Build history of the part. All positions in model axes, mm. A direction names the side the tool comes from. Give positions to 0.01 mm unless a question says otherwise; leave off trailing zeros. Loops run counter-clockwise (first coordinate to the right, second up) from the corner with the lowest first, then second, coordinate; pieces in that order, holes last. Notation, with made-up numbers: M 9,-26.5 L 32,-26.5 A12 ccw 32,-7.5 Z; hole C 13.25,86 d3. An arc over 180 degrees is marked long. Answer in a Markdown table with one row per item. Add a question column.
```python
from build123d import *

# Parameters (mm, degrees)
SKETCH1_W           = 48
SKETCH1_H           = 48
BOSS_EXTRUDE1_DEPTH = 60
SKETCH2_W           = 48
SKETCH2_H           = 48
BOSS_EXTRUDE2_DEPTH = 25
FILLET1_R           = 24
SKETCH3_R           = 5
BOSS_EXTRUDE3_DEPTH = 10
SKETCH4_R           = 5
CUT_EXTRUDE1_DEPTH  = 15
SKETCH5_W           = 31.72674495
SKETCH5_H           = 26.264357258
CUT_EXTRUDE2_DEPTH  = 2
SKETCH8_W           = 31.72674495
SKETCH8_H           = 26.264357258
BOSS_EXTRUDE6_DEPTH = 1
FILLET3_R           = 1.5


# Some blends are built 0.0001 mm under size
with BuildPart() as part:
    # Sketch1 → Boss-Extrude1 (new body)
    with BuildSketch(Plane(origin=(0, 0, 0), x_dir=(1, 0, 0), z_dir=(0, 1, 0))):
        with Locations((24, 24)):
            Rectangle(SKETCH1_W, SKETCH1_H)
    extrude(amount=BOSS_EXTRUDE1_DEPTH)

    # Sketch2 → Boss-Extrude2 (add)
    with BuildSketch(Plane(origin=(48, 0, 0), x_dir=(0, 0, -1), z_dir=(1, 0, 0))):
        with Locations((24, 31.5)):
            Rectangle(SKETCH2_W, SKETCH2_H)
    extrude(amount=BOSS_EXTRUDE2_DEPTH)

    # Fillet1
    fillet1_edges = [part.edges().sort_by_distance(p)[0] for p in [
        (0, 30, 0),
        (0, 30, -48),
        (48, 57.75, -48),
        (48, 57.75, 0),
        (48, 3.75, -48),
        (48, 3.75, 0),
        (60.5, 7.5, 0),
        (60.5, 55.5, 0),
        (60.5, 7.5, -48),
        (60.5, 55.5, -48),
    ]]
    fillet(fillet1_edges, radius=FILLET1_R - 0.0001)  # a hair under: the kernel refuses the full size

    # Sketch3 → Boss-Extrude3 (add)
    with BuildSketch(Plane(origin=(0, 0, 0), x_dir=(-1, 0, 0), z_dir=(0, -1, 0))):
        with Locations(Location((-24, 24, 0), (0, 0, 90))):
            Circle(SKETCH3_R)
    extrude(amount=BOSS_EXTRUDE3_DEPTH)

    # Sketch4 → Cut-Extrude1 (cut)
    with BuildSketch(Plane(origin=(73, 0, 0), x_dir=(0, 0, -1), z_dir=(1, 0, 0))):
        with Locations((24, 31.5)):
            Circle(SKETCH4_R)
    extrude(amount=-CUT_EXTRUDE1_DEPTH, mode=Mode.SUBTRACT)

    # Sketch5 → Cut-Extrude2 (cut)
    with BuildSketch(Plane(origin=(0, 60, 0), x_dir=(1, 0, 0), z_dir=(0, 1, 0))):
        with Locations((23.7045439, 23.7381047)):
            Rectangle(SKETCH5_W, SKETCH5_H)
    extrude(amount=-CUT_EXTRUDE2_DEPTH, mode=Mode.SUBTRACT)

    # Sketch8 → Boss-Extrude6 (add)
    with BuildSketch(Plane(origin=(0, 58, 0), x_dir=(1, 0, 0), z_dir=(0, 1, 0))):
        with Locations((23.7045439, 23.7381047)):
            Rectangle(SKETCH8_W, SKETCH8_H)
    extrude(amount=BOSS_EXTRUDE6_DEPTH)

    # Fillet3
    # the kernel refuses this fillet: 1.5 mm, written as the material it takes off along each edge
    with BuildSketch(Plane(origin=(39.567916375, 60, -10.605926071), x_dir=(0, 0, 1), z_dir=(-1, 0, 0)), Plane(origin=(7.841171425, 60, -36.870283329), x_dir=(0, 0, -1), z_dir=(1, 0, 0))) as fillet3_piece_1:
        with BuildLine():
            CenterArc((1.414213562, -1.5), FILLET3_R, 90, 70.528779366)
            Line((0, -1), (-0.028284271, -0.99))
            ThreePointArc((-0.028284271, -0.99), (-0.03, -0.5), (-0.03, 0))
            Line((-0.03, 0), (0, 0.03))
            Line((0, 0.03), (1.414213562, 0.03))
            Line((1.414213562, 0.03), (1.414213562, 0))
        make_face()
    extrude(amount=31.72674495, mode=Mode.SUBTRACT)
    with BuildSketch(Plane(origin=(39.567916375, 60, -36.870283329), x_dir=(1, 0, 0), z_dir=(0, 0, 1)), Plane(origin=(7.841171425, 60, -10.605926071), x_dir=(-1, 0, 0), z_dir=(0, 0, -1))) as fillet3_piece_2:
        with BuildLine():
            CenterArc((1.414213562, -1.5), FILLET3_R, 90, 70.528779366)
            Line((0, -1), (-0.028284271, -0.99))
            ThreePointArc((-0.028284271, -0.99), (-0.03, -0.5), (-0.03, 0))
            Line((-0.03, 0), (0, 0.03))
            Line((0, 0.03), (1.414213562, 0.03))
            Line((1.414213562, 0.03), (1.414213562, 0))
        make_face()
    extrude(amount=26.264357258, mode=Mode.SUBTRACT)
    with BuildSketch(Plane(origin=(43.103450281, 60, -10.605926071), x_dir=(0, 0, 1), z_dir=(-1, 0, 0))) as fillet3_piece_3a_section:
        with BuildLine():
            CenterArc((1.414213562, -1.5), FILLET3_R, 90, 70.528779366)
            Line((0, -1), (-0.028284271, -0.99))
            ThreePointArc((-0.028284271, -0.99), (-0.03, -0.5), (-0.03, 0))
            Line((-0.03, 0), (0, 0.03))
            Line((0, 0.03), (1.414213562, 0.03))
            Line((1.414213562, 0.03), (1.414213562, 0))
        make_face()
    fillet3_piece_3a = extrude(amount=35.262278856, mode=Mode.PRIVATE)
    fillet3_piece_3a = split(fillet3_piece_3a, bisect_by=Plane(origin=(39.567916375, 59.743234105, -10.266766855), z_dir=(1, 0, 0)), keep=Keep.TOP, mode=Mode.PRIVATE)
    with BuildSketch(Plane(origin=(39.567916375, 60, -36.870283329), x_dir=(1, 0, 0), z_dir=(0, 0, 1))) as fillet3_piece_3b_section:
        with BuildLine():
            CenterArc((1.414213562, -1.5), FILLET3_R, 90, 70.528779366)
            Line((0, -1), (-0.028284271, -0.99))
            ThreePointArc((-0.028284271, -0.99), (-0.03, -0.5), (-0.03, 0))
            Line((-0.03, 0), (0, 0.03))
            Line((0, 0.03), (1.414213562, 0.03))
            Line((1.414213562, 0.03), (1.414213562, 0))
        make_face()
    fillet3_piece_3b = extrude(amount=29.799891164, mode=Mode.PRIVATE)
    fillet3_piece_3b = split(fillet3_piece_3b, bisect_by=Plane(origin=(39.90707559, 59.743234105, -10.605926071), z_dir=(0, 0, 1)), keep=Keep.TOP, mode=Mode.PRIVATE)
    fillet3_piece_3 = fillet3_piece_3a & fillet3_piece_3b
    add(fillet3_piece_3, mode=Mode.SUBTRACT)
    with BuildSketch(Plane(origin=(7.841171425, 60, -7.070392165), x_dir=(-1, 0, 0), z_dir=(0, 0, -1))) as fillet3_piece_4a_section:
        with BuildLine():
            CenterArc((1.414213562, -1.5), FILLET3_R, 90, 70.528779366)
            Line((0, -1), (-0.028284271, -0.99))
            ThreePointArc((-0.028284271, -0.99), (-0.03, -0.5), (-0.03, 0))
            Line((-0.03, 0), (0, 0.03))
            Line((0, 0.03), (1.414213562, 0.03))
            Line((1.414213562, 0.03), (1.414213562, 0))
        make_face()
    fillet3_piece_4a = extrude(amount=29.799891164, mode=Mode.PRIVATE)
    fillet3_piece_4a = split(fillet3_piece_4a, bisect_by=Plane(origin=(7.50201221, 59.743234105, -10.605926071), z_dir=(0, 0, 1)), keep=Keep.TOP, mode=Mode.PRIVATE)
    with BuildSketch(Plane(origin=(39.567916375, 60, -10.605926071), x_dir=(0, 0, 1), z_dir=(-1, 0, 0))) as fillet3_piece_4b_section:
        with BuildLine():
            CenterArc((1.414213562, -1.5), FILLET3_R, 90, 70.528779366)
            Line((0, -1), (-0.028284271, -0.99))
            ThreePointArc((-0.028284271, -0.99), (-0.03, -0.5), (-0.03, 0))
            Line((-0.03, 0), (0, 0.03))
            Line((0, 0.03), (1.414213562, 0.03))
            Line((1.414213562, 0.03), (1.414213562, 0))
        make_face()
    fillet3_piece_4b = extrude(amount=35.262278856, mode=Mode.PRIVATE)
    fillet3_piece_4b = split(fillet3_piece_4b, bisect_by=Plane(origin=(7.841171425, 59.743234105, -10.266766855), z_dir=(-1, 0, 0)), keep=Keep.TOP, mode=Mode.PRIVATE)
    fillet3_piece_4 = fillet3_piece_4a & fillet3_piece_4b
    add(fillet3_piece_4, mode=Mode.SUBTRACT)
    with BuildSketch(Plane(origin=(39.567916375, 60, -40.405817235), x_dir=(1, 0, 0), z_dir=(0, 0, 1))) as fillet3_piece_5a_section:
        with BuildLine():
            CenterArc((1.414213562, -1.5), FILLET3_R, 90, 70.528779366)
            Line((0, -1), (-0.028284271, -0.99))
            ThreePointArc((-0.028284271, -0.99), (-0.03, -0.5), (-0.03, 0))
            Line((-0.03, 0), (0, 0.03))
            Line((0, 0.03), (1.414213562, 0.03))
            Line((1.414213562, 0.03), (1.414213562, 0))
        make_face()
    fillet3_piece_5a = extrude(amount=29.799891164, mode=Mode.PRIVATE)
    fillet3_piece_5a = split(fillet3_piece_5a, bisect_by=Plane(origin=(39.90707559, 59.743234105, -36.870283329), z_dir=(0, 0, -1)), keep=Keep.TOP, mode=Mode.PRIVATE)
    with BuildSketch(Plane(origin=(7.841171425, 60, -36.870283329), x_dir=(0, 0, -1), z_dir=(1, 0, 0))) as fillet3_piece_5b_section:
        with BuildLine():
            CenterArc((1.414213562, -1.5), FILLET3_R, 90, 70.528779366)
            Line((0, -1), (-0.028284271, -0.99))
            ThreePointArc((-0.028284271, -0.99), (-0.03, -0.5), (-0.03, 0))
            Line((-0.03, 0), (0, 0.03))
            Line((0, 0.03), (1.414213562, 0.03))
            Line((1.414213562, 0.03), (1.414213562, 0))
        make_face()
    fillet3_piece_5b = extrude(amount=35.262278856, mode=Mode.PRIVATE)
    fillet3_piece_5b = split(fillet3_piece_5b, bisect_by=Plane(origin=(39.567916375, 59.743234105, -37.209442544), z_dir=(1, 0, 0)), keep=Keep.TOP, mode=Mode.PRIVATE)
    fillet3_piece_5 = fillet3_piece_5a & fillet3_piece_5b
    add(fillet3_piece_5, mode=Mode.SUBTRACT)
    with BuildSketch(Plane(origin=(7.841171425, 60, -10.605926071), x_dir=(-1, 0, 0), z_dir=(0, 0, -1))) as fillet3_piece_6a_section:
        with BuildLine():
            CenterArc((1.414213562, -1.5), FILLET3_R, 90, 70.528779366)
            Line((0, -1), (-0.028284271, -0.99))
            ThreePointArc((-0.028284271, -0.99), (-0.03, -0.5), (-0.03, 0))
            Line((-0.03, 0), (0, 0.03))
            Line((0, 0.03), (1.414213562, 0.03))
            Line((1.414213562, 0.03), (1.414213562, 0))
        make_face()
    fillet3_piece_6a = extrude(amount=29.799891164, mode=Mode.PRIVATE)
    fillet3_piece_6a = split(fillet3_piece_6a, bisect_by=Plane(origin=(7.50201221, 59.743234105, -36.870283329), z_dir=(0, 0, -1)), keep=Keep.TOP, mode=Mode.PRIVATE)
    with BuildSketch(Plane(origin=(4.305637519, 60, -36.870283329), x_dir=(0, 0, -1), z_dir=(1, 0, 0))) as fillet3_piece_6b_section:
        with BuildLine():
            CenterArc((1.414213562, -1.5), FILLET3_R, 90, 70.528779366)
            Line((0, -1), (-0.028284271, -0.99))
            ThreePointArc((-0.028284271, -0.99), (-0.03, -0.5), (-0.03, 0))
            Line((-0.03, 0), (0, 0.03))
            Line((0, 0.03), (1.414213562, 0.03))
            Line((1.414213562, 0.03), (1.414213562, 0))
        make_face()
    fillet3_piece_6b = extrude(amount=35.262278856, mode=Mode.PRIVATE)
    fillet3_piece_6b = split(fillet3_piece_6b, bisect_by=Plane(origin=(7.841171425, 59.743234105, -37.209442544), z_dir=(-1, 0, 0)), keep=Keep.TOP, mode=Mode.PRIVATE)
    fillet3_piece_6 = fillet3_piece_6a & fillet3_piece_6b
    add(fillet3_piece_6, mode=Mode.SUBTRACT)


solid = part.part
```
(1) Slice it at D-D, the plane x = 20. Give the cut face in (y, z), then the cut area to 3 significant figures.
(2) Wall check: line 1 (Y direction, x = 68, z = -24); line 2 (Z direction, x = 46, y = 31); line 3 (Y direction, x = 5.5, z = -20). Give the ranges that are in metal, low to high.
(3) Pull direction Z, two halves, no side cores. Call faces 1 (the cylindrical face through (37.55, 8.97, -43.81)), 2 (the flat face through (24, 0, -30)), 3 (the flat face through (23, 59, -24)): +Z half, -Z half, draft (parallel to the pull), parting line (faces both ways), or undercut.
(4) Tool access for faces 4 (the flat face through (58, 32, -24)), 5 (the cylindrical face through (54.29, 45.05, -43.81)), 6 (the cylindrical face through (37.55, 8.97, -4.19)), 7 (the cylindrical face through (19.12, -4.93, -22.92)): list every direction of +Z, -Z, +X, -X, +Y, -Y with a clear straight run to the whole face (end or side of a thin tool).
(5) Pin check, flat tips, straight feed: pin 1 (3 mm diameter, centred on x = 59.5, z = -7, fed in from -Y); pin 2 (10 mm diameter, centred on x = 60, z = -6, fed in from -Y); pin 3 (10 mm diameter, centred on x = 16, z = -7.5, fed in from -Y). Stop position of each tip, or through.
(6) Slice it at B-B, the plane z = -26. Give the cut face in (x, y), then the cut area to 3 significant figures.
Solution:
| question | item | result |
|---|---|---|
| 1 | outline | M -10,-27 L 0,-27 L 0,-47.66 L 60,-47.66 L 60,-38.28 A1.5 ccw 59,-36.87 L 59,-10.61 A1.5 ccw 60,-9.19 L 60,-0.34 L 0,-0.34 L 0,-21 L -10,-21 Z |
| 1 | area | 2,870 mm^2 |
| 2 | line 1 | 7.5 to 26.5, 36.5 to 55.5 |
| 2 | line 2 | -47.99 to -0.01 |
| 2 | line 3 | 0 to 60 |
| 3 | face 1 | -Z half |
| 3 | face 2 | draft |
| 3 | face 3 | undercut |
| 4 | face 4 | +X |
| 4 | face 5 | -Z, +X, +Y |
| 4 | face 6 | +Z, +X, -Y |
| 4 | face 7 | -Y |
| 5 | pin 1 | y = 13.18 |
| 5 | pin 2 | y = 11.33 |
| 5 | pin 3 | y = 0 |
| 6 | outline | M 0.08,0 L 19.42,0 L 19.42,-10 L 28.58,-10 L 28.58,0 L 47.92,0 L 47.92,7.58 L 73,7.58 L 73,26.92 L 58,26.92 L 58,36.08 L 73,36.08 L 73,55.42 L 47.92,55.42 L 47.92,60 L 40.98,60 A1.5 ccw 39.57,59 L 7.84,59 A1.5 ccw 6.43,60 L 0.08,60 Z |
| 6 | area | 3,990 mm^2 |
